Verification items for the finished model (mm, model axes). A direction names the side the tool comes from. Coordinates: 2 decimals unless noted, no trailing zeros. Write each loop counter-clockwise with the first axis right and the second up, starting at its lowest first coordinate (ties: lowest second). Pieces come first, ordered by that corner, then holes. Notation, with made-up numbers: (-34.75, -13.5) -> (-29.75, -13.5) arc R20 cw to (-29.75, 25.5) -> close; hole circle Ø6 at (59, -19.5). An arc over 180 degrees is marked (long way). Use CSV: the item, a comma, the result in double quotes.
```python
from build123d import *

# Parameters (mm, degrees)
F0_W     = 87
F0_H     = 7.4
F0_R     = 3
F1_DEPTH = 3.95
F0_R_2   = 2.499
F2_DEPTH = 2.95
F3_R     = 3.69999


# Not quite as in the source:
# - a fillet or chamfer is up to 0.001 mm smaller than in the source, because OpenCascade refuses the exact size


with BuildPart() as f1:
    # F0 (on Front) → F1 (new body, symmetric)
    with BuildSketch(Plane.XZ):
        Rectangle(F0_W, F0_H)
        with Locations((-40, 0)):
            Circle(F0_R, mode=Mode.SUBTRACT)
        with Locations((-32, 0)):
            Circle(F0_R, mode=Mode.SUBTRACT)
        with Locations((-24, 0)):
            Circle(F0_R, mode=Mode.SUBTRACT)
        with Locations((-16, 0)):
            Circle(F0_R, mode=Mode.SUBTRACT)
        with Locations((-8, 0)):
            Circle(F0_R, mode=Mode.SUBTRACT)
        Circle(F0_R, mode=Mode.SUBTRACT)
        with Locations((8, 0)):
            Circle(F0_R, mode=Mode.SUBTRACT)
        with Locations((16, 0)):
            Circle(F0_R, mode=Mode.SUBTRACT)
        with Locations((24, 0)):
            Circle(F0_R, mode=Mode.SUBTRACT)
        with Locations((32, 0)):
            Circle(F0_R, mode=Mode.SUBTRACT)
        with Locations((40, 0)):
            Circle(F0_R, mode=Mode.SUBTRACT)
    extrude(amount=F1_DEPTH, both=True)

    # F0 (on Front) → F2 (join, symmetric)
    with BuildSketch(Plane.XZ):
        with Locations((-40, 0)):
            Circle(F0_R)
        with Locations((-40, 0)):
            Circle(F0_R_2, mode=Mode.SUBTRACT)
        with Locations((-32, 0)):
            Circle(F0_R)
        with Locations((-32, 0)):
            Circle(F0_R_2, mode=Mode.SUBTRACT)
        with Locations((-24, 0)):
            Circle(F0_R)
        with Locations((-24, 0)):
            Circle(F0_R_2, mode=Mode.SUBTRACT)
        with Locations((-16, 0)):
            Circle(F0_R)
        with Locations((-16, 0)):
            Circle(F0_R_2, mode=Mode.SUBTRACT)
        with Locations((-8, 0)):
            Circle(F0_R)
        with Locations((-8, 0)):
            Circle(F0_R_2, mode=Mode.SUBTRACT)
        Circle(F0_R)
        Circle(F0_R_2, mode=Mode.SUBTRACT)
        with Locations((8, 0)):
            Circle(F0_R)
        with Locations((8, 0)):
            Circle(F0_R_2, mode=Mode.SUBTRACT)
        with Locations((16, 0)):
            Circle(F0_R)
        with Locations((16, 0)):
            Circle(F0_R_2, mode=Mode.SUBTRACT)
        with Locations((24, 0)):
            Circle(F0_R)
        with Locations((24, 0)):
            Circle(F0_R_2, mode=Mode.SUBTRACT)
        with Locations((32, 0)):
            Circle(F0_R)
        with Locations((32, 0)):
            Circle(F0_R_2, mode=Mode.SUBTRACT)
        with Locations((40, 0)):
            Circle(F0_R)
        with Locations((40, 0)):
            Circle(F0_R_2, mode=Mode.SUBTRACT)
    extrude(amount=F2_DEPTH, both=True)

    # F3 (radius 3.7 in the source; OpenCascade refuses exactly that, so slightly less here)
    f3_edges = [f1.edges().sort_by_distance(p)[0] for p in [
        (-43.5, 0, 3.7),
        (-43.5, 0, -3.7),
        (43.5, 0, 3.7),
        (43.5, 0, -3.7),
    ]]
    fillet(f3_edges, radius=F3_R)


solid = f1.part
```
1) Mould release check, pull along X, two halves, no side actions. Record for faces 1 (the flat face through (-1, -3.95, -3)), 2 (the cylindrical face through (37, -3.4, 0.1)): released by +X, released by -X, zero draft, split by the parting line, or undercut.
Return value:
face 1,"zero draft"
face 2,"undercut"
2) Scan lines: L1, parallel to Z at x = -24, y = 1.25; L2, parallel to Z at x = 40, y = 3.5; L3, parallel to Y at x = -30.5, z = 2.5. Record each from-to range of solid material in increasing order.
Return value:
L1,"-3.7 to -2.5, 2.5 to 3.7"
L2,"-3.69 to -3, 3 to 3.69"
L3,"-2.95 to 2.95"
3) Cross-section at A-A (x = 24). Record the boundary of the cut face in (y, z).
Return value:
outline,"(-3.95, -3.7) -> (3.95, -3.7) -> (3.95, -3) -> (2.95, -3) -> (2.95, -2.5) -> (-2.95, -2.5) -> (-2.95, -3) -> (-3.95, -3) -> close; (-3.95, 3) -> (-2.95, 3) -> (-2.95, 2.5) -> (2.95, 2.5) -> (2.95, 3) -> (3.95, 3) -> (3.95, 3.7) -> (-3.95, 3.7) -> close"
4) Set-up check for faces 3 (the cylindrical face through (10.77, 3.46, -1.15)), 4 (the cylindrical face through (-35, -3.4, 0.1)), 5 (the flat face through (-1, 3.95, -3)): record each of +Z, -Z, +X, -X, +Y, -Y from which the full face is reachable in a straight line by a thin tool's end or side.
Return value:
face 3,"+Y"
face 4,"-Y"
face 5,"+Z, -Z, +X, -X, +Y"
5) Cross-section at C-C (x = 33). Record the boundary of the cut face in (y, z).
Return value:
outline,"(-3.95, -3.7) -> (3.95, -3.7) -> (3.95, -2.83) -> (2.95, -2.83) -> (2.95, -2.29) -> (-2.95, -2.29) -> (-2.95, -2.83) -> (-3.95, -2.83) -> close; (-3.95, 2.83) -> (-2.95, 2.83) -> (-2.95, 2.29) -> (2.95, 2.29) -> (2.95, 2.83) -> (3.95, 2.83) -> (3.95, 3.7) -> (-3.95, 3.7) -> close"
6) Cross-section at B-B (y = 0.75). Give the number of separate pieces and of enclosed holes in the cut face, plus the area to 3 significant figures.
Return value:
separate pieces,"1"
enclosed holes,"11"
area,"416 mm2"
7) Gauge pin test, flat ends, axial feed: pin 1 (2 mm diameter, centred on x = -7, z = -0.5, fed in from -Y); pin 2 (4 mm diameter, centred on y = 3, z = 2, fed in from +X). Record the tip position at first contact, or that the pin passes through.
Return value:
pin 1,"through"
pin 2,"x = 43.5"
